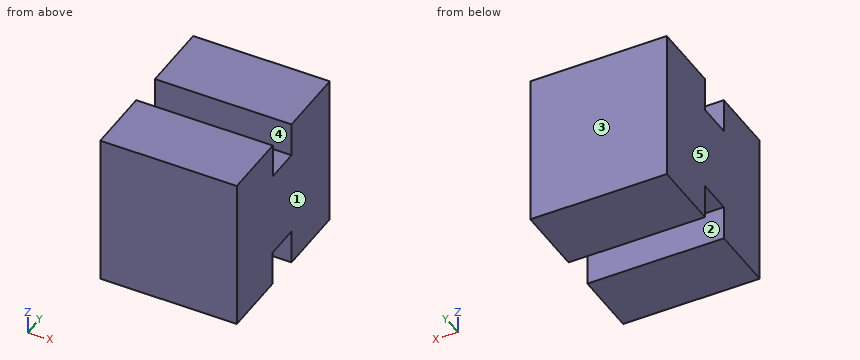
from build123d import *

# Parameters (mm, degrees)
F0_W     = 50.9128235281
F0_H     = 63.8054171577
F1_DEPTH = 57.15
F2_W     = 12.8643363714
F2_H     = 12.7601113558
F3_DEPTH = 76.2
F4_W     = 12.8961652517
F4_H     = 12.868527323
F5_DEPTH = 76.2


with BuildPart() as f1:
    # F0 (on Top) → F1 (new body)
    with BuildSketch(Plane.XY):
        with Locations((-62.0051566511, 23.6927601509)):
            Rectangle(F0_W, F0_H)
    extrude(amount=F1_DEPTH)

    # F2 (on face) → F3 (cut)
    with BuildSketch(Plane(origin=(-87.4615684152, 0, 0), x_dir=(0, -1, 0), z_dir=(-1, 0, 0))):
        with Locations((-22.8889267892, 50.7699443221)):
            Rectangle(F2_W, F2_H)
    extrude(amount=-F3_DEPTH, mode=Mode.SUBTRACT)

    # F4 (on face) → F5 (cut)
    with BuildSketch(Plane(origin=(-87.4615684152, 0, 0), x_dir=(0, -1, 0), z_dir=(-1, 0, 0))):
        with Locations((-22.873012349, 6.4342636615)):
            Rectangle(F4_W, F4_H)
    extrude(amount=-F5_DEPTH, mode=Mode.SUBTRACT)


solid = f1.part
Source: CAD feature listing. Evaluate the final solid. Frame: model axes, mm. Face numbers are marked on the shaded views. A direction names the side the tool comes from. Give positions to 0.01 mm unless a question says otherwise; leave off trailing zeros. Loops run counter-clockwise (first coordinate to the right, second up) from the corner with the lowest first, then second, coordinate; pieces in that order, holes last. Notation, with made-up numbers: (9, 46.25) -> (44, 46.25) arc R23 cw to (44, 69.25) -> close; hole circle Ø2 at (83, 63.25). An arc over 180 degrees is marked (long way). Use a Markdown table: item, result. Add a question column.
1) Line query: line 1 along Y through (x, z) = (-54, 53); line 2 along Z through (x, y) = (-72, 19). Output: solid intervals per line, ascending. Write a range as [from, to].
2) Reachability of the marked faces 1 and 2 from +Z, -Z, +X, -X, +Y, -Y: full face, straight path, thin tool, end or side. Return the list, or none.
3) Section query A-A, the plane z = 4.5. Return the cut outline in (x, y), then the cut area to 3 significant figures.
4) Section query B-B, the plane x = -41. Return the cut outline in (y, z).
5) Pull-direction query (Y, two-part tool) for the marked faces 3, 4 and 5; classes: +Y half, -Y half, draft (parallel to the pull), parting line (faces both ways), or undercut.
6) First-contact query: pin 1 (4 mm diameter, centred on x = -50, y = 23.5, fed in from -Z). Flat tip, straight axial feed; report the tip coordinate or a pass-through.
7) Section query C-C, the plane y = 17.5. Return the cut outline in (x, z).
Numbers:
| question | item | result |
|---|---|---|
| 1 | line 1 | y = [-8.21, 16.46], [29.32, 55.6] |
| 1 | line 2 | z = [12.87, 44.39] |
| 2 | face 1 | +Z, -Z, +X, +Y, -Y |
| 2 | face 2 | -Z, +X, -X |
| 3 | outline | (-87.46, -8.21) -> (-36.55, -8.21) -> (-36.55, 16.42) -> (-87.46, 16.42) -> close; (-87.46, 29.32) -> (-36.55, 29.32) -> (-36.55, 55.6) -> (-87.46, 55.6) -> close |
| 3 | area | 2,590 mm2 |
| 4 | outline | (-8.21, 0) -> (16.42, 0) -> (16.42, 12.87) -> (29.32, 12.87) -> (29.32, 0) -> (55.6, 0) -> (55.6, 57.15) -> (29.32, 57.15) -> (29.32, 44.39) -> (16.46, 44.39) -> (16.46, 57.15) -> (-8.21, 57.15) -> close |
| 5 | face 3 | +Y half |
| 5 | face 4 | undercut |
| 5 | face 5 | draft |
| 6 | pin 1 | stops at z = 12.87 |
| 7 | outline | (-87.46, 12.87) -> (-36.55, 12.87) -> (-36.55, 44.39) -> (-87.46, 44.39) -> close |
